```python
from build123d import *
from build123d import SkipClean  # not in build123d's __all__

# Parameters (mm, degrees)
F1_DEPTH = 25.4
F3_DEPTH = 12.7
F4_DEPTH = 6.35
F5_DEPTH = 31.75


# Not quite as in the source:
# - after a boolean that leaves OpenCascade's solid faulty, fix() repairs it


with BuildPart() as f1:
    # F0 (on Top) → F1 (new body)
    with BuildSketch(Plane.XY):
        with BuildLine():
            ThreePointArc((22.225, -150.7707178964), (115.3534784911, -99.5958583476), (152.4, 0))
            ThreePointArc((152.4, 0), (149.696971962, 28.5758041952), (141.6837718451, 56.1379443491))
            ThreePointArc((141.6837718451, 56.1379443491), (131.9822715367, 76.2), (119.4587718451, 94.6327735473))
            ThreePointArc((119.4587718451, 94.6327735473), (28.5758041952, 149.696971962), (-76.2, 131.9822715367))
            ThreePointArc((-76.2, 131.9822715367), (-99.5958583476, 115.3534784911), (-119.4587718451, 94.6327735473))
            ThreePointArc((-119.4587718451, 94.6327735473), (-131.9822715367, 76.2), (-141.6837718451, 56.1379443491))
            ThreePointArc((-141.6837718451, 56.1379443491), (-143.9292826863, -50.1011136144), (-76.2, -131.9822715367))
            ThreePointArc((-76.2, -131.9822715367), (-50.1011136144, -143.9292826863), (-22.225, -150.7707178964))
            ThreePointArc((-22.225, -150.7707178964), (0, -152.4), (22.225, -150.7707178964))
        make_face()
    extrude(amount=F1_DEPTH)

    # F2 (on face) → F3 (cut)
    with BuildSketch(Plane.XY.offset(25.4)):
        with BuildLine():
            ThreePointArc((22.225, -72.8868257986), (61.2371823323, -45.3480705212), (76.2, 0))
            ThreePointArc((76.2, 0), (75.7069908166, 8.6539899179), (74.2343427428, 17.1959983002))
            ThreePointArc((74.2343427428, 17.1959983002), (65.9911357684, 38.1), (52.0093427428, 55.6908274984))
            ThreePointArc((52.0093427428, 55.6908274984), (0, 76.2), (-52.0093427428, 55.6908274984))
            ThreePointArc((-52.0093427428, 55.6908274984), (-65.9911357684, 38.1), (-74.2343427428, 17.1959983002))
            ThreePointArc((-74.2343427428, 17.1959983002), (-65.9911357684, -38.1), (-22.225, -72.8868257986))
            ThreePointArc((-22.225, -72.8868257986), (0, -76.2), (22.225, -72.8868257986))
        make_face()
    extrude(amount=-F3_DEPTH, mode=Mode.SUBTRACT)

    # F2 (on face) → F4 (join)
    with BuildSketch(Plane.XY.offset(25.4)):
        with BuildLine():
            ThreePointArc((-74.2343427428, 17.1959983002), (-65.9911357684, 38.1), (-52.0093427428, 55.6908274984))
            Line((-52.0093427428, 55.6908274984), (-119.4587718451, 94.6327735473))
            ThreePointArc((-119.4587718451, 94.6327735473), (-131.9822715367, 76.2), (-141.6837718451, 56.1379443491))
            Line((-141.6837718451, 56.1379443491), (-74.2343427428, 17.1959983002))
        make_face()
        with BuildLine():
            Line((22.225, -150.7707178964), (22.225, -72.8868257986))
            ThreePointArc((22.225, -72.8868257986), (0, -76.2), (-22.225, -72.8868257986))
            Line((-22.225, -72.8868257986), (-22.225, -150.7707178964))
            ThreePointArc((-22.225, -150.7707178964), (0, -152.4), (22.225, -150.7707178964))
        make_face()
        with BuildLine():
            ThreePointArc((52.0093427428, 55.6908274984), (65.9911357684, 38.1), (74.2343427428, 17.1959983002))
            Line((74.2343427428, 17.1959983002), (141.6837718451, 56.1379443491))
            ThreePointArc((141.6837718451, 56.1379443491), (131.9822715367, 76.2), (119.4587718451, 94.6327735473))
            Line((119.4587718451, 94.6327735473), (52.0093427428, 55.6908274984))
        make_face()
    with SkipClean():  # cleaning this boolean's faces spoils the solid; the shape is the same uncleaned
        extrude(amount=F4_DEPTH)

    # F0 (on Top) → F5 (join)
    with BuildSketch(Plane.XY):
        with BuildLine():
            ThreePointArc((119.4587718451, 94.6327735473), (131.9822715367, 76.2), (141.6837718451, 56.1379443491))
            Line((141.6837718451, 56.1379443491), (174.9637268225, 75.3521353139))
            ThreePointArc((174.9637268225, 75.3521353139), (164.9778394209, 95.25), (152.7387268225, 113.8469645122))
            Line((152.7387268225, 113.8469645122), (119.4587718451, 94.6327735473))
        make_face()
        with BuildLine():
            ThreePointArc((-141.6837718451, 56.1379443491), (-131.9822715367, 76.2), (-119.4587718451, 94.6327735473))
            Line((-119.4587718451, 94.6327735473), (-152.7387268225, 113.8469645122))
            ThreePointArc((-152.7387268225, 113.8469645122), (-164.9778394209, 95.25), (-174.9637268225, 75.3521353139))
            Line((-174.9637268225, 75.3521353139), (-141.6837718451, 56.1379443491))
        make_face()
        with BuildLine():
            Line((22.225, -189.1990998261), (22.225, -150.7707178964))
            ThreePointArc((22.225, -150.7707178964), (0, -152.4), (-22.225, -150.7707178964))
            Line((-22.225, -150.7707178964), (-22.225, -189.1990998261))
            ThreePointArc((-22.225, -189.1990998261), (0, -190.5), (22.225, -189.1990998261))
        make_face()
    extrude(amount=F5_DEPTH)

    add(f1.part.fix(), mode=Mode.REPLACE)


solid = f1.part
```
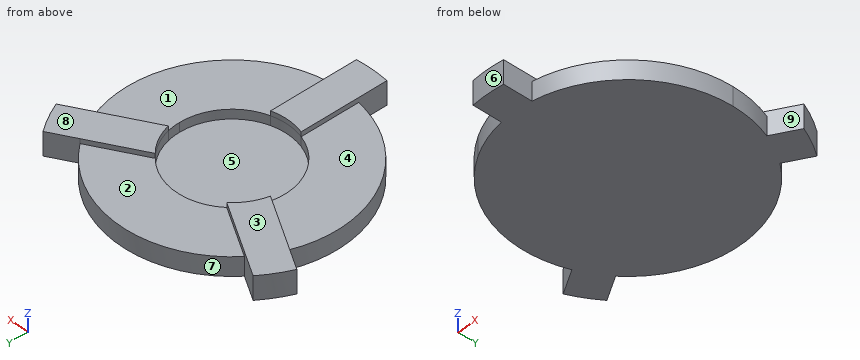
Geometry check sheet. Reference: the model listing, model coordinates, mm. Face numbers are marked on the shaded views. A direction names the side the tool comes from. Give positions to 0.01 mm unless a question says otherwise; leave off trailing zeros. Write each loop counter-clockwise with the first axis right and the second up, starting at its lowest first coordinate (ties: lowest second). Pieces come first, ordered by that corner, then holes. Notation, with made-up numbers: (-10.5, 60) -> (26.5, 60) arc R22 cw to (26.5, 80) -> close; hole circle Ø7 at (-10, 26.5). An arc over 180 degrees is marked (long way). Use one line per item in the form item = value.
Item 1: Mould release check, pull along Y, two halves, no side actions. Record for the marked faces 6, 7, 8 and 9: released by +Y, released by -Y, zero draft, split by the parting line, or undercut.
Results list:
face_6 = released by -Y
face_7 = released by +Y
face_8 = zero draft
face_9 = undercut
Item 2: Sectioned sample at C-C on y = -67. Enter the section's corners in (x, z), plus the area to 3 significant figures.
Results list:
outline = (-136.88, 0) -> (136.88, 0) -> (136.88, 25.4) -> (36.3, 25.4) -> (36.3, 12.7) -> (-36.3, 12.7) -> (-36.3, 25.4) -> (-136.88, 25.4) -> close
area = 6,030 mm2
Item 3: Access from +Z, -Z, +X, -X, +Y, -Y to the whole of each face (thin tool, end or side, straight path). Record for the marked faces 1, 2, 3, 4 and 5.
Results list:
face_1 = +Z, +X, -Y
face_2 = +Z, +Y
face_3 = +Z, +X, -X, +Y, -Y
face_4 = +Z, -X, -Y
face_5 = +Z
Item 4: Sectioned sample at D-D on y = -165. Enter the section's corners in (x, z) (3 decimals).
Results list:
outline = (-22.225, 0) -> (22.225, 0) -> (22.225, 31.75) -> (-22.225, 31.75) -> close
Item 5: Sectioned sample at A-A on x = 85. Enter the section's corners in (y, z), plus the area to 3 significant figures.
Results list:
outline = (-126.49, 0) -> (126.49, 0) -> (126.49, 25.4) -> (74.74, 25.4) -> (74.74, 31.75) -> (23.41, 31.75) -> (23.41, 25.4) -> (-126.49, 25.4) -> close
area = 6,750 mm2
Item 6: Scan lines: line 1 (X direction, y = 100, z = 19); line 2 (Z direction, x = 35, y = 21); line 3 (Z direction, x = -130, y = -52). Record each from-to range of solid material in increasing order.
Results list:
line_1 = -162.14 to -128.76, -115 to 115, 128.76 to 162.14
line_2 = 0 to 12.7
line_3 = 0 to 25.4
Item 7: Sectioned sample at B-B on z = 7. Enter the section's corners in (x, y) (3 decimals).
Results list:
outline = (-174.964, 75.352) -> (-141.684, 56.138) arc R152.4 ccw to (-22.225, -150.771) -> (-22.225, -189.199) arc R190.5 ccw to (22.225, -189.199) -> (22.225, -150.771) arc R152.4 ccw to (141.684, 56.138) -> (174.964, 75.352) arc R190.5 ccw to (152.739, 113.847) -> (119.459, 94.633) arc R152.4 ccw to (-119.459, 94.633) -> (-152.739, 113.847) arc R190.5 ccw to start
Item 8: Depth check by flat-ended pin: pin 1 Ø2 at (y, z) = (105.5, 9.5) entering from -X; pin 2 Ø8 at (x, z) = (-17.5, 10.5) entering from +Y; pin 3 Ø1.5 at (x, z) = (-49.5, 3.5) entering from +Y. Enter the tip coordinate at first touch or a pass-through.
Results list:
pin_1 = -159.28
pin_2 = 151.8
pin_3 = 144.39
